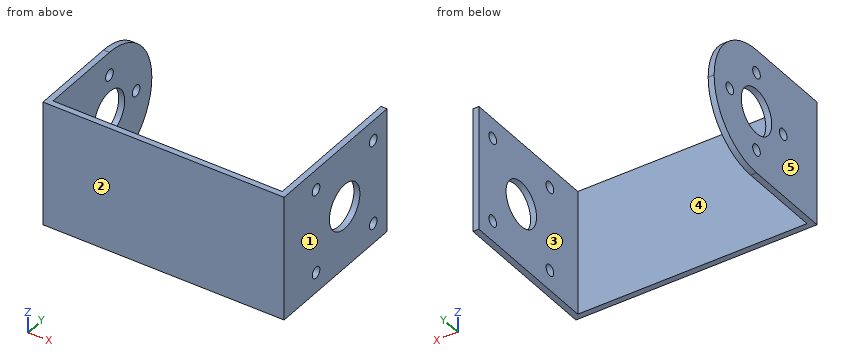
from build123d import *

# Parameters (mm, degrees)
BOSS_EXTRUDE1_DEPTH = 22.225
FILLET1_R           = 11.1125
SKETCH3_R           = 4
SKETCH3_R_2         = 1
CUT_EXTRUDE2_DEPTH  = 1.058333333
CIRPATTERN1_COUNT   = 4
CUT_EXTRUDE3_START  = -1.058333333
SKETCH2_R           = 1
SKETCH2_R_2         = 4
CUT_EXTRUDE3_DEPTH  = 1.058333333


with BuildPart() as part:
    # Sketch1 → Boss-Extrude1 (new body)
    with BuildSketch(Plane.XY):
        Polygon((0, 26.9875), (0, 0), (42.8625, 0), (42.8625, 26.9875), (41.804166667, 26.9875), (41.804166667, 1.058333333), (1.058333333, 1.058333333), (1.058333333, 26.9875), align=None)
    extrude(amount=BOSS_EXTRUDE1_DEPTH)

    # Fillet1
    fillet1_edges = [part.edges().sort_by_distance(p)[0] for p in [
        (0.529166667, 26.9875, 0),
        (0.529166667, 26.9875, 22.225),
    ]]
    fillet(fillet1_edges, radius=FILLET1_R - 0.0001)  # a hair under: the kernel refuses the full size

    # Sketch3 → Cut-Extrude2 (cut)
    with BuildSketch(Plane.ZY):
        with Locations((11.1125, 15.875)):
            Circle(SKETCH3_R)
        with Locations((11.1125, 22.875)):
            Circle(SKETCH3_R_2)
    cut_extrude2 = extrude(amount=-CUT_EXTRUDE2_DEPTH, mode=Mode.SUBTRACT)

    # CirPattern1: Cut-Extrude2 ×4 about axis
    cirpattern1_axis = Axis((0, 15.875, 11.1125), (1, 0, 0))
    for i in range(1, CIRPATTERN1_COUNT):
        add(cut_extrude2.rotate(cirpattern1_axis, i * 360 / CIRPATTERN1_COUNT), mode=Mode.SUBTRACT)

    # Sketch2 → Cut-Extrude3 (cut)
    with BuildSketch(Plane(origin=(42.8625, 0, 0), x_dir=(0, 0, -1), z_dir=(1, 0, 0)).offset(CUT_EXTRUDE3_START)):
        with Locations((-3.6125, 23.375)):
            Circle(SKETCH2_R)
        with Locations((-18.6125, 23.375)):
            Circle(SKETCH2_R)
        with Locations((-3.6125, 8.375)):
            Circle(SKETCH2_R)
        with Locations((-18.6125, 8.375)):
            Circle(SKETCH2_R)
        with Locations(Location((-11.1125, 15.875, 0), (0, 0, 180))):
            Circle(SKETCH2_R_2)
    extrude(amount=CUT_EXTRUDE3_DEPTH, mode=Mode.SUBTRACT)


solid = part.part
The listing builds one solid part. Answer for the finished solid, in the listing's coordinates (mm). Face numbers are marked on the shaded views. A direction names the side the tool comes from. Coordinates: 2 decimals unless noted, no trailing zeros. Loops run counter-clockwise (first coordinate to the right, second up) from the corner with the lowest first, then second, coordinate; pieces in that order, holes last.
1) Find the intervals of material crossed by L1, parallel to X at y = 2.5, z = 15.25; L2, parallel to Y at x = 5.5, z = 6.25, in increasing order.
2) Find section A-A on y = 12.75. Write down the section's boundary in (x, z) (1 decimal), then the cut area to 3 significant figures.
3) Determine the mould class of the marked faces 1, 2 and 3 for opening direction X: pulls with the +X half, pulls with the -X half, needs draft (parallel to the pull), parting line crosses it, or undercut.
4) Flat-ended cylindrical pins translate along their axes: pin 1 Ø6.5 at (y, z) = (13.5, 14) entering from -X; pin 2 Ø12 at (x, z) = (22.5, 18) entering from +Y. Find the tip coordinate at first contact, or state that the pin passes through.
5) Find section B-B on z = 8. Write down the section's boundary in (x, y), then the cut area to 3 significant figures.
6) Find section D-D on z = 1.5. Write down the section's boundary in (x, y).
7) Find section C-C on x = 14. Write down the section's boundary in (y, z) (3 decimals), then the cut area to 3 significant figures.
8) A tool of negligible diameter and unlimited length cuts with its end or side. For the marked faces 4 and 5, from which of +Z, -Z, +X, -X, +Y, -Y can it reach the whole face along a straight path? Write none if from no direction.
Values:
1. L1: x = 0 to 1.06, 41.8 to 42.86
1. L2: y = 0 to 1.06
2. outline: (0, 0) - (1.1, 0) - (1.1, 8.6) - (0, 8.6) - close; (0, 13.6) - (1.1, 13.6) - (1.1, 22.2) - (0, 22.2) - close; (41.8, 0) - (42.9, 0) - (42.9, 8.6) - (41.8, 8.6) - close; (41.8, 13.6) - (42.9, 13.6) - (42.9, 22.2) - (41.8, 22.2) - close
2. area: 36.5 mm2
3. face 1: pulls with the +X half
3. face 2: needs draft
3. face 3: undercut
4. pin 1: stops at x = 0
4. pin 2: stops at y = 1.06
5. outline: (0, 0) - (42.86, 0) - (42.86, 13.36) - (41.8, 13.36) - (41.8, 1.06) - (1.06, 1.06) - (1.06, 13.36) - (0, 13.36) - close; (0, 18.39) - (1.06, 18.39) - (1.06, 26.54) - (0, 26.54) - close; (41.8, 18.39) - (42.86, 18.39) - (42.86, 26.99) - (41.8, 26.99) - close
5. area: 89.1 mm2
6. outline: (0, 0) - (42.86, 0) - (42.86, 26.99) - (41.8, 26.99) - (41.8, 1.06) - (1.06, 1.06) - (1.06, 21.45) - (0, 21.45) - close
7. outline: (0, 0) - (1.058, 0) - (1.058, 22.225) - (0, 22.225) - close
7. area: 23.5 mm2
8. face 4: +Z, -Z, +Y
8. face 5: +Z, -Z, -X, +Y, -Y
